The model under review builds one solid part; all positions refer to its coordinate system, in mm. Face numbers are marked on the shaded views. A direction names the side the tool comes from. Coordinates: 2 decimals unless noted, no trailing zeros. Order: outer loops, then holes, each group sorted by start corner. A loop starts at its lowest first (then second) coordinate and runs counter-clockwise, first axis right, second up. Notation, with made-up numbers: M -6,55 L 1,55 A24 ccw 1,92 Z; hole C 56.25,77 d11. An arc over 180 degrees is marked long. One line per item, written item: value.
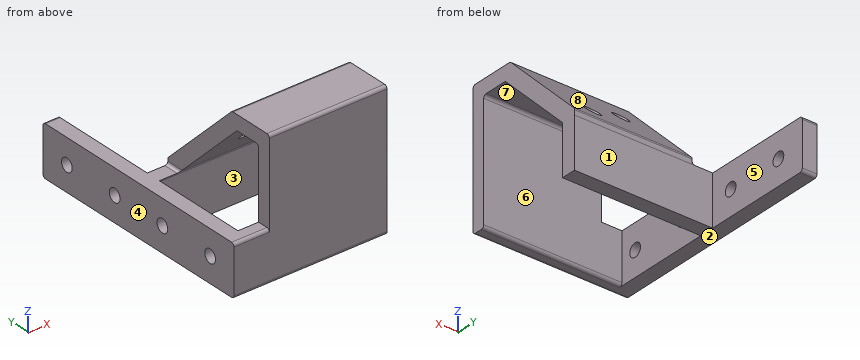
```python
from build123d import *
from build123d.topology import SkipClean

# Parameters (mm, degrees)
SKETCH1_W           = 17
SKETCH1_H           = 80
BOSS_EXTRUDE1_DEPTH = 5
SKETCH2_R           = 2.25
CUT_EXTRUDE1_DEPTH  = 82.939001702
SKETCH3_W           = 17
SKETCH3_H           = 5
SKETCH3_H_2         = 4.5
BOSS_EXTRUDE2_DEPTH = 7
BOSS_EXTRUDE3_DEPTH = 40
CUT_EXTRUDE2_REACH  = 89.054
SKETCH6_R           = 2.75
FILLET1_START       = 5
FILLET1_DEPTH       = 48
FILLET1_START_2     = -1
FILLET1_2_DEPTH     = 13
FILLET1_START_3     = 10.9999999
FILLET1_3_DEPTH     = 4.7752001
FILLET1_START_4     = 12
FILLET1_4_DEPTH     = 40
FILLET1_5_DEPTH     = 12
FILLET1_6_DEPTH     = 43.5
FILLET1_7_DEPTH     = 16.909322952


with BuildPart() as part:
    # Sketch1 → Boss-Extrude1 (new body)
    with BuildSketch(Plane(origin=(0, 0, 0), x_dir=(0, 0, -1), z_dir=(1, 0, 0))):
        with Locations((8.5, 40)):
            Rectangle(SKETCH1_W, SKETCH1_H)
    extrude(amount=BOSS_EXTRUDE1_DEPTH)

    # Sketch2 → Cut-Extrude1 (cut, through all)
    with BuildSketch(Plane(origin=(5, 0, 0), x_dir=(0, 0, -1), z_dir=(1, 0, 0))):
        with Locations((8.5, 10)):
            Circle(SKETCH2_R)
        with Locations((8.5, 30)):
            Circle(SKETCH2_R)
        with Locations((8.5, 50)):
            Circle(SKETCH2_R)
        with Locations((8.5, 70)):
            Circle(SKETCH2_R)
    extrude(amount=-CUT_EXTRUDE1_DEPTH, mode=Mode.SUBTRACT)

    # Sketch3 → Boss-Extrude2 (add)
    with BuildSketch(Plane(origin=(5, 0, 0), x_dir=(0, 0, -1), z_dir=(1, 0, 0))):
        with Locations((8.5, 40)):
            Rectangle(SKETCH3_W, SKETCH3_H)
        with Locations((8.5, 2.25)):
            Rectangle(SKETCH3_W, SKETCH3_H_2)
    extrude(amount=BOSS_EXTRUDE2_DEPTH)

    # Sketch5 → Boss-Extrude3 (add)
    with BuildSketch(Plane(origin=(12, 0, 0), x_dir=(0, 0, -1), z_dir=(1, 0, 0))):
        Polygon((0, 37.5), (-23.954638078, 13.545361922), (-23.954638078, 4.5), (17, 4.5), (17, 0), (-28.954638078, 0), (-28.954638078, 5), (-28.954638078, 15.616429734), (-2.084580393, 42.486487419), (0, 42.5), (17, 42.5), (17, 37.5), align=None)
    extrude(amount=BOSS_EXTRUDE3_DEPTH)

    # Sketch6 → Cut-Extrude2 (cut, up to next)
    with BuildSketch(Plane(origin=(0, 22.285533906, 22.285533906), x_dir=(1, 0, 0), z_dir=(0, 0.7071067811865482, 0.7071067811865468)), mode=Mode.PRIVATE) as cut_extrude2_sk1:
        with Locations(Location((40.25, 18.818462431, 0), (0, 0, 270))):
            Circle(SKETCH6_R)
    cut_extrude2_tool1 = extrude(cut_extrude2_sk1.sketch, amount=-CUT_EXTRUDE2_REACH, mode=Mode.PRIVATE) & part.part
    # Sketch6 → Cut-Extrude2 (cut, up to next)
    with BuildSketch(Plane(origin=(0, 22.285533906, 22.285533906), x_dir=(1, 0, 0), z_dir=(0, 0.7071067811865482, 0.7071067811865468)), mode=Mode.PRIVATE) as cut_extrude2_sk2:
        with Locations(Location((24.25, 7.718462431, 0), (0, 0, 270))):
            Circle(SKETCH6_R)
    cut_extrude2_tool2 = extrude(cut_extrude2_sk2.sketch, amount=-CUT_EXTRUDE2_REACH, mode=Mode.PRIVATE) & part.part
    add(cut_extrude2_tool1.solids().sort_by_distance((40.25, 35.592196, 8.978872))[0], mode=Mode.SUBTRACT)
    add(cut_extrude2_tool2.solids().sort_by_distance((24.25, 27.743311, 16.827757))[0], mode=Mode.SUBTRACT)

    # Fillet1: read off the stored shape, not the designer's step
    # Fillet1 outline → Fillet1 (cut)
    with BuildSketch(Plane.YZ.offset(FILLET1_START)):
        with BuildLine():
            Line((4.5, -17), (4.5, -16))
            ThreePointArc((4.5, -16), (4.207106781, -16.707106781), (3.5, -17))
            Line((3.5, -17), (4.5, -17))
        make_face()
        with BuildLine():
            Line((0, -17), (1, -17))
            ThreePointArc((1, -17), (0.292893219, -16.707106781), (0, -16))
            Line((0, -16), (0, -17))
        make_face()
        with BuildLine():
            Line((0, 28.954638078), (0, 27.954638078))
            ThreePointArc((0, 27.954638078), (0.292893219, 28.661744859), (1, 28.954638078))
            Line((1, 28.954638078), (0, 28.954638078))
        make_face()
        with BuildLine():
            ThreePointArc((42.19627557, 2.374792242), (42.411803181, 2.053361203), (42.48914778, 1.674167483))
            Line((42.48914778, 1.674167483), (42.486487419, 2.084580393))
            Line((42.486487419, 2.084580393), (42.19627557, 2.374792242))
        make_face()
        with BuildLine():
            Line((15.616429734, 28.954638078), (15.202216171, 28.954638078))
            ThreePointArc((15.202216171, 28.954638078), (15.584899604, 28.878517611), (15.909322952, 28.661744859))
            Line((15.909322952, 28.661744859), (15.616429734, 28.954638078))
        make_face()
    extrude(amount=FILLET1_DEPTH, mode=Mode.SUBTRACT)

    # Fillet1 2 outline → Fillet1 2 (cut)
    with BuildSketch(Plane.YZ.offset(FILLET1_START_2)):
        with BuildLine():
            Line((0, -17), (1, -17))
            ThreePointArc((1, -17), (0.292893219, -16.707106781), (0, -16))
            Line((0, -16), (0, -17))
        make_face()
        with BuildLine():
            ThreePointArc((0, -1), (0.292893219, -0.292893219), (1, 0))
            Line((1, 0), (0, 0))
            Line((0, 0), (0, -1))
        make_face()
        with BuildLine():
            ThreePointArc((80, -16), (79.707106781, -16.707106781), (79, -17))
            Line((79, -17), (80, -17))
            Line((80, -17), (80, -16))
        make_face()
        with BuildLine():
            Line((80, 0), (79, 0))
            ThreePointArc((79, 0), (79.707106781, -0.292893219), (80, -1))
            Line((80, -1), (80, 0))
        make_face()
    extrude(amount=FILLET1_2_DEPTH, mode=Mode.SUBTRACT)

    # Fillet1 3 outline → Fillet1 3 (add)
    with SkipClean():  # the faces are left unmerged after this step: merging them gives an invalid solid
        with BuildSketch(Plane.YZ.offset(FILLET1_START_3)):
            with BuildLine():
                Line((4.5, 0), (4.5, 23.954638078))
                Line((4.5, 23.954638078), (13.545361922, 23.954638078))
                Line((13.545361922, 23.954638078), (37.207106781, 0.292893219))
                ThreePointArc((37.207106781, 0.292893219), (37.423879533, -0.03153013), (37.5, -0.414213562))
                Line((37.5, -0.414213562), (37.5, 0))
                Line((37.5, 0), (42.5, 0))
                Line((42.5, 0), (42.48914778, 1.674167483))
                ThreePointArc((42.48914778, 1.674167483), (42.411803181, 2.053361203), (42.19627557, 2.374792242))
                Line((42.19627557, 2.374792242), (15.909322952, 28.661744859))
                ThreePointArc((15.909322952, 28.661744859), (15.584899604, 28.878517611), (15.202216171, 28.954638078))
                Line((15.202216171, 28.954638078), (1, 28.954638078))
                ThreePointArc((1, 28.954638078), (0.292893219, 28.661744859), (0, 27.954638078))
                Line((0, 27.954638078), (0, 0))
                Line((0, 0), (4.5, 0))
            make_face()
        extrude(amount=FILLET1_3_DEPTH)
    add(part.part.scale(1), mode=Mode.REPLACE)  # the faces are merged on a copy

    # Fillet1 4 outline → Fillet1 4 (add)
    with BuildSketch(Plane.YZ.offset(FILLET1_START_4)):
        with BuildLine():
            Line((37.5, -0.414213562), (37.5, 0))
            Line((37.5, 0), (37.207106781, 0.292893219))
            ThreePointArc((37.207106781, 0.292893219), (37.423879533, -0.03153013), (37.5, -0.414213562))
        make_face()
        with BuildLine():
            Line((4.5, 23.954638078), (4.5, 22.954638078))
            ThreePointArc((4.5, 22.954638078), (4.792893219, 23.661744859), (5.5, 23.954638078))
            Line((5.5, 23.954638078), (4.5, 23.954638078))
        make_face()
        with BuildLine():
            ThreePointArc((13.131148359, 23.954638078), (13.513831792, 23.878517611), (13.838255141, 23.661744859))
            Line((13.838255141, 23.661744859), (13.545361922, 23.954638078))
            Line((13.545361922, 23.954638078), (13.131148359, 23.954638078))
        make_face()
    extrude(amount=FILLET1_4_DEPTH)

    # Fillet1 5 outline → Fillet1 5 (add)
    with BuildSketch(Plane.YZ):
        with BuildLine():
            Line((37.5, 0), (37.410179722, 0))
            ThreePointArc((37.410179722, 0), (37.47728699, -0.202293437), (37.5, -0.414213562))
            Line((37.5, -0.414213562), (37.5, 0))
        make_face()
    extrude(amount=FILLET1_5_DEPTH)

    # Fillet1 6 outline → Fillet1 6 (cut)
    with BuildSketch(Plane(origin=(0, 0, 0), x_dir=(1, 0, 0), z_dir=(0, 1, 0)).offset(FILLET1_START_2)):
        with BuildLine():
            Line((10.9999999, -28.954638078), (12, -28.954638078))
            Line((12, -28.954638078), (12, -1))
            ThreePointArc((12, -1), (11.707106781, -0.292893219), (11, 0))
            Line((11, 0), (10.9999999, -28.954638078))
        make_face()
    extrude(amount=FILLET1_6_DEPTH, mode=Mode.SUBTRACT)

    # Fillet1 7 outline → Fillet1 7 (cut)
    with BuildSketch(Plane(origin=(0, 0, 0), x_dir=(1, 0, 0), z_dir=(0, 1, 0)).offset(FILLET1_START_2)):
        with BuildLine():
            Line((12, 0), (11, 0))
            ThreePointArc((11, 0), (11.707106781, -0.292893219), (12, -1))
            Line((12, -1), (12, 0))
        make_face()
    extrude(amount=FILLET1_7_DEPTH, mode=Mode.SUBTRACT)


solid = part.part
```
(1) For L1, parallel to Y at x = 2, z = -8.5; L2, parallel to Y at x = 30.5, z = 17.5; L3, parallel to Y at x = 36, z = 5.5, list the stretches that pass through material, from the lowest coordinate up.
Geometry results:
L1: y = 0 to 7.75, 12.25 to 27.75, 32.25 to 47.75, 52.25 to 67.75, 72.25 to 80
L2: y = 0 to 4.5, 20 to 27.07
L3: y = 0 to 4.5, 32 to 39.07
(2) We need section A-A, the plane y = 10. State the section outline as (x, z) points, plus the area to 4 significant figures.
Geometry results:
outline: M 0,-17 L 5,-17 L 5,-10.75 L 0,-10.75 Z; M 0,-6.25 L 5,-6.25 L 5,0 L 0,0 Z; M 12,23.95 L 52,23.95 L 52,28.95 L 12,28.95 Z
area: 262.5 mm2
(3) Insertion check: pin 1 Ø12 at (x, z) = (45.5, 4) entering from +Y; pin 2 Ø8.5 at (x, y) = (40.5, 10) entering from -Z; pin 3 Ø13.5 at (y, z) = (28.5, -9) entering from +X. Each pin has a flat end and moves straight along its axis. Give the tip position at first contact, or say it passes through.
Geometry results:
pin 1: stops at y = 42.5
pin 2: stops at z = 23.25
pin 3: stops at x = 5
(4) We need section B-B, the plane z = -8.5. State the section outline as (x, y) points.
Geometry results:
outline: M 0,0 L 52,0 L 52,4.5 L 5,4.5 L 5,7.75 L 0,7.75 Z; M 0,12.25 L 5,12.25 L 5,27.75 L 0,27.75 Z; M 0,32.25 L 5,32.25 L 5,37.5 L 52,37.5 L 52,42.5 L 5,42.5 L 5,47.75 L 0,47.75 Z; M 0,52.25 L 5,52.25 L 5,67.75 L 0,67.75 Z; M 0,72.25 L 5,72.25 L 5,80 L 0,80 Z
(5) We need section C-C, the plane x = 45. State the section outline as (y, z) points, plus the area to 3 significant figures.
Geometry results:
outline: M 0,-16 A1 ccw 1,-17 L 3.5,-17 A1 ccw 4.5,-16 L 4.5,22.95 A1 cw 5.5,23.95 L 13.13,23.95 A1 cw 13.84,23.66 L 37.21,0.29 A1 cw 37.5,-0.41 L 37.5,-17 L 42.5,-17 L 42.5,0 L 42.49,1.67 A1 ccw 42.2,2.37 L 15.91,28.66 A1 ccw 15.2,28.95 L 1,28.95 A1 ccw 0,27.95 Z
area: 527 mm2
(6) We need section D-D, the plane y = 70. State the section outline as (x, z) points, plus the area to 3 significant figures.
Geometry results:
outline: M 0,-17 L 5,-17 L 5,-10.75 L 0,-10.75 Z; M 0,-6.25 L 5,-6.25 L 5,0 L 0,0 Z
area: 62.5 mm2
(7) Tool access review of the marked faces 4, 5, 6, 7 and 8: name each direction out of +Z, -Z, +X, -X, +Y, -Y from which nothing blocks a thin tool from reaching the whole face with its end or side.
Geometry results:
face 4: +Z, -Z, -X, +Y, -Y
face 5: +Z, -Z, +X, +Y
face 6: -Z, +X
face 7: -Z, +X, -X
face 8: +Z, +X, -X, +Y
(8) Mouldability with a two-part tool opening along Y and no side actions: class the marked faces 1, 2 and 3 as +Y half, -Y half, draft (parallel to the pull), parting line (faces both ways), or undercut.
Geometry results:
face 1: +Y half
face 2: draft
face 3: undercut
